from build123d import *

# Parameters (mm, degrees)
BASE_FLANGE1_DEPTH            = 22
CUT_EXTRUDE1_DEPTH            = 62.294881516
CUT_EXTRUDE1_DEPTH_BACK       = 62.294881516
EDGE_FLANGE3_STRIP_W          = 6.5232
EDGE_FLANGE3_STRIP_H          = 1.25
EDGE_FLANGE3_STRIP_CUT_DEPTH  = 31
EDGE_FLANGE3_RELIEF_W         = 7.1482
EDGE_FLANGE3_RELIEF_H         = 0.625
EDGE_FLANGE3_RELIEF_CUT_DEPTH = 1.25
EDGE_FLANGE3_DEPTH            = 31
CUT_EXTRUDE2_DEPTH            = 62.773396377


# Read off the part's stored shape, not the designer's step: Base-Flange1
# Sheet-metal steps are written as plain solids
with BuildPart() as part:
    # Base-Flange1 outline → Base-Flange1 (new body)
    with BuildSketch(Plane.XY):
        with BuildLine():
            Line((-51.19559942, 14.5), (11, 14.5))
            Line((11, 14.5), (11, 15.75))
            Line((11, 15.75), (-51.19559942, 15.75))
            ThreePointArc((-51.19559942, 15.75), (-52.404310309, 15.339977796), (-53.114079989, 14.279163381))
            ThreePointArc((-53.114079989, 14.279163381), (-55, 0), (-53.114079989, -14.279163381))
            ThreePointArc((-53.114079989, -14.279163381), (-52.404310309, -15.339977796), (-51.19559942, -15.75))
            Line((-51.19559942, -15.75), (11, -15.75))
            Line((11, -15.75), (11, -14.5))
            Line((11, -14.5), (-51.19559942, -14.5))
            ThreePointArc((-51.19559942, -14.5), (-51.643770386, -14.347970223), (-51.906941808, -13.954636941))
            ThreePointArc((-51.906941808, -13.954636941), (-53.75, 0), (-51.906941808, 13.954636941))
            ThreePointArc((-51.906941808, 13.954636941), (-51.643770386, 14.347970223), (-51.19559942, 14.5))
        make_face()
    extrude(amount=BASE_FLANGE1_DEPTH)

    # Sketch2 → Cut-Extrude1 (cut, two sides: drawn at the far end of the back side and taken through both)
    with BuildSketch(Plane(origin=(0, 0, 0), x_dir=(1, 0, 0), z_dir=(0, 1, 0)).offset(-CUT_EXTRUDE1_DEPTH_BACK)):
        with BuildLine():
            Line((8.3, -11.5), (-4.2, -11.5))
            ThreePointArc((-4.2, -11.5), (-5.7, -13), (-4.2, -14.5))
            Line((-4.2, -14.5), (8.3, -14.5))
            ThreePointArc((8.3, -14.5), (9.8, -13), (8.3, -11.5))
        make_face()
        with BuildLine():
            Line((8.3, 14.5), (-4.2, 14.5))
            ThreePointArc((-4.2, 14.5), (-5.7, 13), (-4.2, 11.5))
            Line((-4.2, 11.5), (8.3, 11.5))
            ThreePointArc((8.3, 11.5), (9.8, 13), (8.3, 14.5))
        make_face()
    extrude(amount=CUT_EXTRUDE1_DEPTH + CUT_EXTRUDE1_DEPTH_BACK, mode=Mode.SUBTRACT)

    # Edge-Flange3 strip (across the edge) → Edge-Flange3 strip cut (cut)
    with BuildSketch(Plane(origin=(11, 14.5, 22.05), x_dir=(0, 0, -1), z_dir=(-1, 0, 0))):
        with Locations((-2.525, -0.625)):
            Rectangle(EDGE_FLANGE3_STRIP_W, EDGE_FLANGE3_STRIP_H)
    extrude(amount=EDGE_FLANGE3_STRIP_CUT_DEPTH, mode=Mode.SUBTRACT)

    # Edge-Flange3 relief (on the sheet) → Edge-Flange3 relief cut (cut)
    with BuildSketch(Plane(origin=(11, 14.5, 21.3134), x_dir=(0, 0, -1), z_dir=(0, -1, 0))):
        with Locations((-2.9491, -31.3125)):
            Rectangle(EDGE_FLANGE3_RELIEF_W, EDGE_FLANGE3_RELIEF_H)
    extrude(amount=-EDGE_FLANGE3_RELIEF_CUT_DEPTH, mode=Mode.SUBTRACT)

    # Edge-Flange3 section (across the edge) → Edge-Flange3 (add)
    with BuildSketch(Plane(origin=(11, 14.5, 22.05), x_dir=(0, 0, -1), z_dir=(-1, 0, 0))):
        with BuildLine():
            Line((-1.25, 0.7366), (-1.25, 28.95))
            Line((-1.25, 28.95), (0, 28.95))
            Line((0, 28.95), (0, 0.7366))
            ThreePointArc((0, 0.7366), (0.215745145, 0.215745145), (0.7366, 0))
            Line((0.7366, 0), (0.7366, -1.25))
            ThreePointArc((0.7366, -1.25), (-0.668138332, -0.668138332), (-1.25, 0.7366))
        make_face()
    extrude(amount=EDGE_FLANGE3_DEPTH)

    # Sketch29 → Cut-Extrude2 (cut, through all)
    with BuildSketch(Plane.XY.offset(23.3)):
        with BuildLine():
            Line((8.3, -6.25), (-4.2, -6.25))
            ThreePointArc((-4.2, -6.25), (-5.7, -7.75), (-4.2, -9.25))
            Line((-4.2, -9.25), (8.3, -9.25))
            ThreePointArc((8.3, -9.25), (9.8, -7.75), (8.3, -6.25))
        make_face()
        with BuildLine():
            Line((8.3, 6.25), (-4.2, 6.25))
            ThreePointArc((-4.2, 6.25), (-5.7, 7.75), (-4.2, 9.25))
            Line((-4.2, 9.25), (8.3, 9.25))
            ThreePointArc((8.3, 9.25), (9.8, 7.75), (8.3, 6.25))
        make_face()
    extrude(amount=-CUT_EXTRUDE2_DEPTH, mode=Mode.SUBTRACT)

    # Mirror1: part across plane


with BuildPart() as part_1:
    add(part.part)
    add(part.part.mirror(Plane(origin=(-51.906941808, -13.954636941, 0), x_dir=(1, 0, 0), z_dir=(0, 0, -1))))


solid = part_1.part
Read the model definition and answer for the solid it produces. Units are mm, in the model's axes. A direction names the side the tool comes from. Give positions to 0.01 mm unless a question says otherwise; leave off trailing zeros. Loops run counter-clockwise (first coordinate to the right, second up) from the corner with the lowest first, then second, coordinate; pieces in that order, holes last. Notation, with made-up numbers: M 78.25,73 L 120.25,73 A16 ccw 120.25,85 Z; hole C 20.5,21.5 d9. An arc over 180 degrees is marked long. Write each question's results on one line, items separated by ' | '.
1. Section A-A on z = -13 is taken. Give the vertices of the cut face in (x, y), plus the area to 3 significant figures.
Values:
outline: M -53.11,-14.28 A1.99 ccw -51.2,-15.75 L -5.7,-15.75 L -5.7,-14.5 L -51.2,-14.5 A0.74 cw -51.91,-13.95 A53.75 cw -51.91,13.95 A0.74 cw -51.2,14.5 L -5.7,14.5 L -5.7,15.75 L -51.2,15.75 A1.99 ccw -53.11,14.28 A55 ccw Z; M 9.8,-15.75 L 11,-15.75 L 11,-14.5 L 9.8,-14.5 Z; M 9.8,14.5 L 11,14.5 L 11,15.75 L 9.8,15.75 Z | area: 157 mm^2
2. A tool of negligible diameter and unlimited length cuts with its end or side. For faces 5 (the face through (9.8, -7.8, 22.7)), 6 (the face through (9.8, -15.1, -13)), 7 (the face through (-4, 0, 23.3)), from which of +Z, -Z, +X, -X, +Y, -Y can it reach the whole face along a straight path? Write none if from no direction.
Values:
face 5: +Z, -Z | face 6: +Y, -Y | face 7: +Z, +X, -X, +Y, -Y
3. The mould has two halves that part along X. Classify faces 1 (the face through (11, 15, 0)), 2 (the face through (-52.39, 15.35, 0.31)), 3 (the face through (-20, 15.75, 0)), 4 (the face through (9.8, -7.8, -22.7)): pulls with the +X half, pulls with the -X half, needs draft (parallel to the pull), parting line crosses it, or undercut.
Values:
face 1: pulls with the +X half | face 2: pulls with the -X half | face 3: needs draft | face 4: undercut
4. Section B-B on x = -16 is taken. Give the vertices of the cut face in (y, z), plus the area to 3 significant figures.
Values:
outline: M -15.75,-22 L -14.5,-22 L -14.5,22 L -15.75,22 Z; M -14.45,-23.3 L 13.76,-23.3 A1.99 ccw 15.75,-21.31 L 15.75,21.31 A1.99 ccw 13.76,23.3 L -14.45,23.3 L -14.45,22.05 L 13.76,22.05 A0.74 cw 14.5,21.31 L 14.5,-21.31 A0.74 cw 13.76,-22.05 L -14.45,-22.05 Z | area: 184 mm^2
5. Given pin 1 (3 mm diameter, centred on y = 5.5, z = 22.5, fed in from -X); pin 2 (1.4 mm diameter, centred on x = -0.5, y = 15, fed in from +Z); pin 3 (0.6 mm diameter, centred on x = -0.5, z = 22.5, fed in from +Y); pin 4 (3 mm diameter, centred on x = -43, y = 12.5, fed in from +Z), each flat-ended and moving along its own axis, determine where each tip first touches the part or whether it passes through.
Values:
pin 1: stops at x = -54.85 | pin 2: stops at z = 23.23 | pin 3: stops at y = 15.54 | pin 4: passes through
6. Section C-C on y = 8.5 is taken. Give the vertices of the cut face in (x, z).
Values:
outline: M -54.34,-22 L -53.07,-22 L -53.07,22 L -54.34,22 Z; M -20,-23.3 L -5.5,-23.3 L -5.5,-22.05 L -20,-22.05 Z; M -20,22.05 L -5.5,22.05 L -5.5,23.3 L -20,23.3 Z; M 9.6,-23.3 L 11,-23.3 L 11,-22.05 L 9.6,-22.05 Z; M 9.6,22.05 L 11,22.05 L 11,23.3 L 9.6,23.3 Z
7. Straight lines are drawn through the part: line 1 (Y direction, x = -23, z = -14.5); line 2 (Z direction, x = -7, y = -12.5); line 3 (X direction, y = 0.5, z = -12). For each, find the intervals that lie inside material, in ascending order. Write a range as [from, to].
Values:
line 1: y = [-15.75, -14.5], [14.5, 15.75] | line 2: z = [-23.3, -22.05], [22.05, 23.3] | line 3: x = [-55, -53.75]
8. Section D-D on y = 2 is taken. Give the vertices of the cut face in (x, z).
Values:
outline: M -54.96,-22 L -53.71,-22 L -53.71,22 L -54.96,22 Z; M -20,-23.3 L 11,-23.3 L 11,-22.05 L -20,-22.05 Z; M -20,22.05 L 11,22.05 L 11,23.3 L -20,23.3 Z
